from build123d import *

# Parameters (mm, degrees)
SKETCH1_W                                    = 27
SKETCH1_H                                    = 46
SKETCH1_R                                    = 1.75
BOSS_EXTRUDE1_DEPTH                          = 1
SKETCH2_R                                    = 3
SKETCH2_R_2                                  = 1.75
SKETCH2_R_3                                  = 2.25
BOSS_EXTRUDE2_DEPTH                          = 5
SKETCH3_R                                    = 3.5
CUT_EXTRUDE1_DEPTH                           = 3
CHAMFER1_SIZE                                = 2
CHAMFER1_SIZE2                               = 0.5
CHAMFER1_PART_2_SIZE                         = 2
CHAMFER1_PART_2_SIZE2                        = 0.5
CHAMFER2_SIZE                                = 0.5
CSK_FOR_M3_FLAT_COUNTERSUNK_HEAD_SCR_2_COUNT = 2
CSK_FOR_M3_FLAT_COUNTERSUNK_HEAD_SCR_2_PITCH = 35.302266216
CSK_FOR_M3_FLAT_COUNTERSUNK_HEAD_SCR_3_COUNT = 2
CSK_FOR_M3_FLAT_COUNTERSUNK_HEAD_SCR_3_PITCH = 35.302266216
FILLET1_R                                    = 2


with BuildPart() as part:
    # Sketch1 → Boss-Extrude1 (new body, symmetric)
    with BuildSketch(Plane.XY):
        Rectangle(SKETCH1_W, SKETCH1_H)
        Circle(SKETCH1_R, mode=Mode.SUBTRACT)
        with Locations((0, 17)):
            Circle(SKETCH1_R, mode=Mode.SUBTRACT)
        with Locations((-9.5, -17)):
            Circle(SKETCH1_R, mode=Mode.SUBTRACT)
        with Locations((9.5, -17)):
            Circle(SKETCH1_R, mode=Mode.SUBTRACT)
        with BuildLine():
            Line((-3.25, 13), (3.25, 13))
            ThreePointArc((3.25, 13), (5.194543648, 12.194543648), (6, 10.25))
            Line((6, 10.25), (6, 7.75))
            ThreePointArc((6, 7.75), (5.194543648, 5.805456352), (3.25, 5))
            Line((3.25, 5), (-3.25, 5))
            ThreePointArc((-3.25, 5), (-5.194543648, 5.805456352), (-6, 7.75))
            Line((-6, 7.75), (-6, 10.25))
            ThreePointArc((-6, 10.25), (-5.194543648, 12.194543648), (-3.25, 13))
        make_face(mode=Mode.SUBTRACT)
        with BuildLine():
            Line((-3.25, -5), (3.25, -5))
            ThreePointArc((3.25, -5), (5.194543648, -5.805456352), (6, -7.75))
            Line((6, -7.75), (6, -10.25))
            ThreePointArc((6, -10.25), (5.194543648, -12.194543648), (3.25, -13))
            Line((3.25, -13), (-3.25, -13))
            ThreePointArc((-3.25, -13), (-5.194543648, -12.194543648), (-6, -10.25))
            Line((-6, -10.25), (-6, -7.75))
            ThreePointArc((-6, -7.75), (-5.194543648, -5.805456352), (-3.25, -5))
        make_face(mode=Mode.SUBTRACT)
    extrude(amount=BOSS_EXTRUDE1_DEPTH, both=True)

    # Sketch2 → Boss-Extrude2 (add)
    with BuildSketch(Plane.XY.offset(1)):
        Circle(SKETCH2_R)
        Circle(SKETCH2_R_2, mode=Mode.SUBTRACT)
        with Locations((-9, 0)):
            Circle(SKETCH2_R_3)
        with Locations((7.5, 0)):
            Circle(SKETCH2_R_3)
    extrude(amount=BOSS_EXTRUDE2_DEPTH)

    # Sketch3 → Cut-Extrude1 (cut)
    with BuildSketch(Plane.XY.offset(6)):
        Circle(SKETCH3_R)
    extrude(amount=-CUT_EXTRUDE1_DEPTH, mode=Mode.SUBTRACT)

    # Chamfer1
    chamfer1_edges = [part.edges().sort_by_distance(p)[0] for p in [
        (-11.25, 0, 6),
    ]]
    chamfer1_side = [part.faces().sort_by_distance(p)[0] for p in [
        (-11.25, 0, 3.5),
    ]]
    chamfer(chamfer1_edges, length=CHAMFER1_SIZE, length2=CHAMFER1_SIZE2, reference=chamfer1_side[0])

    # Chamfer1 part 2
    chamfer1_part_2_edges = [part.edges().sort_by_distance(p)[0] for p in [
        (5.25, 0, 6),
    ]]
    chamfer1_part_2_side = [part.faces().sort_by_distance(p)[0] for p in [
        (5.25, 0, 3.5),
    ]]
    chamfer(chamfer1_part_2_edges, length=CHAMFER1_PART_2_SIZE, length2=CHAMFER1_PART_2_SIZE2, reference=chamfer1_part_2_side[0])

    # Chamfer2
    chamfer2_edges = [part.edges().sort_by_distance(p)[0] for p in [
        (-3, 0, 3),
    ]]
    chamfer(chamfer2_edges, length=CHAMFER2_SIZE)

    # Sketch5 → CSK for M3 Flat Countersunk Head Screw1 (revolve, cut)
    with BuildSketch(Plane(origin=(0, 17, 1), x_dir=(0, -1, 0), z_dir=(1, 0, 0))):
        Polygon((0, 0), (0, 2), (1.7, 2), (1.7, 1.65), (3.35, 0), align=None)
    csk_for_m3_flat_countersunk_head_screw1 = revolve(axis=Axis((0, 17, 7.35), (0, 0, -1)), mode=Mode.SUBTRACT)

    # CSK for M3 Flat Countersunk Head Scr 2: CSK for M3 Flat Countersunk Head Screw1 ×2
    with Locations(*[Vector(-0.269104537, -0.963110974, 0) * (i * CSK_FOR_M3_FLAT_COUNTERSUNK_HEAD_SCR_2_PITCH) for i in range(1, CSK_FOR_M3_FLAT_COUNTERSUNK_HEAD_SCR_2_COUNT)]):
        add(csk_for_m3_flat_countersunk_head_screw1, mode=Mode.SUBTRACT)

    # CSK for M3 Flat Countersunk Head Scr 3: CSK for M3 Flat Countersunk Head Screw1 ×2
    with Locations(*[Vector(0.269104537, -0.963110974, 0) * (i * CSK_FOR_M3_FLAT_COUNTERSUNK_HEAD_SCR_3_PITCH) for i in range(1, CSK_FOR_M3_FLAT_COUNTERSUNK_HEAD_SCR_3_COUNT)]):
        add(csk_for_m3_flat_countersunk_head_screw1, mode=Mode.SUBTRACT)

    # Fillet1
    fillet1_edges = [part.edges().sort_by_distance(p)[0] for p in [
        (-13.5, 23, 0),
        (13.5, 23, 0),
        (13.5, -23, 0),
        (-13.5, -23, 0),
    ]]
    fillet(fillet1_edges, radius=FILLET1_R)


solid = part.part
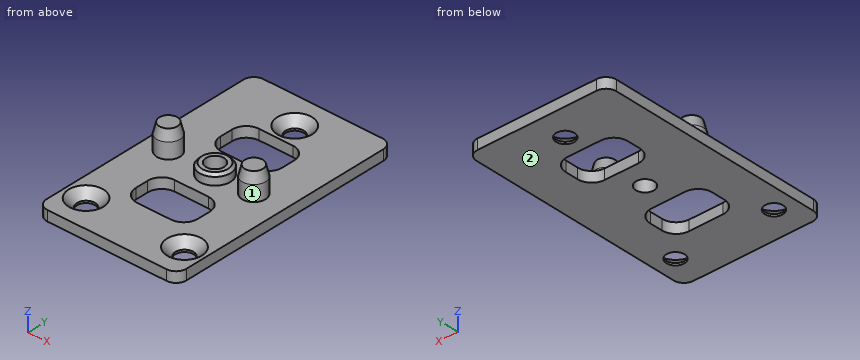
Part model, mm, in its own coordinate system. Face numbers are marked on the shaded views. Give positions to 0.01 mm unless a question says otherwise; leave off trailing zeros. Write each loop counter-clockwise with the first axis right and the second up, starting at its lowest first coordinate (ties: lowest second). Pieces come first, ordered by that corner, then holes.
1) Cut at A-A on y = -9.5. Write the cut outline in (x, z), then the cut area to 3 significant figures.
Resolved:
outline: (-13.5, -1) - (-6, -1) - (-6, 1) - (-13.5, 1) - close; (6, -1) - (13.5, -1) - (13.5, 1) - (6, 1) - close
area: 30.0 mm2
2) Cut at D-D on y = 17. Write the cut outline in (x, z), then the cut area to 3 significant figures.
Resolved:
outline: (-13.5, -1) - (-1.75, -1) - (-1.75, -0.6) - (-3.35, 1) - (-13.5, 1) - close; (1.75, -1) - (13.5, -1) - (13.5, 1) - (3.35, 1) - (1.75, -0.6) - close
area: 44.4 mm2
3) Two-plate mould, pull along X, no slides. Class the marked faces 1 and 2: released by +X, released by -X, zero draft, split by the parting line, or undercut.
Resolved:
face 1: undercut
face 2: zero draft
4) Probe L1, parallel to X at y = -17, z = -0.85; L2, parallel to Y at x = 0, z = -0.8; L3, parallel to Y at x = 9.5, z = -0.8. List the from-to ranges inside material, lowest first.
Resolved:
L1: x = -13.5 to -11.25, -7.75 to 7.75, 11.25 to 13.5
L2: y = -23 to -13, -5 to -1.75, 1.75 to 5, 13 to 15.25, 18.75 to 23
L3: y = -23 to -18.75, -15.25 to 23
5) Cut at B-B on x = 0. Write the cut outline in (y, z).
Resolved:
outline: (-23, -1) - (-13, -1) - (-13, 1) - (-23, 1) - close; (-5, -1) - (-1.75, -1) - (-1.75, 3) - (-2.5, 3) - (-3, 2.5) - (-3, 1) - (-5, 1) - close; (1.75, -1) - (5, -1) - (5, 1) - (3, 1) - (3, 2.5) - (2.5, 3) - (1.75, 3) - close; (13, -1) - (15.25, -1) - (15.25, -0.6) - (13.65, 1) - (13, 1) - close; (18.75, -1) - (23, -1) - (23, 1) - (20.35, 1) - (18.75, -0.6) - close
6) Cut at C-C on z = 3.5. Write the cut outline in (x, y).
Resolved:
outline: circle Ø4.5 at (-9, 0); circle Ø4.5 at (7.5, 0)
7) Pin check, flat tips, straight feed: pin 1 (10 mm diameter, centred on x = 5, y = -11.5, fed in from +Z); pin 2 (3 mm diameter, centred on x = -9.5, z = 4.5, fed in from +Y); pin 3 (2 mm diameter, centred on x = 0, y = 0, fed in from +Z); pin 4 (1.5 mm diameter, centred on x = 1, y = 0.5, fed in from +Z). Stop position of each tip, or through.
Resolved:
pin 1: stops at z = 1
pin 2: stops at y = 2.25
pin 3: passes through
pin 4: stops at z = 3
